Source: CAD feature listing. Evaluate the final solid. Frame: model axes, mm. A direction names the side the tool comes from. Give positions to 0.01 mm unless a question says otherwise; leave off trailing zeros. Loops run counter-clockwise (first coordinate to the right, second up) from the corner with the lowest first, then second, coordinate; pieces in that order, holes last. Notation, with made-up numbers: (79, 35) - (114, 35) arc R14 cw to (114, 57) - close; hole circle Ø7 at (1, 50.5). An arc over 180 degrees is marked (long way). Put each result on its own line as item: value.
```python
from build123d import *

# Parameters (mm, degrees)
F1_DEPTH = 152.4
F3_DEPTH = 151.892


with BuildPart() as f1:
    # F0 (on Top) → F1 (new body)
    with BuildSketch(Plane.XY):
        Polygon((127, 0), (0, 0), (-127, 0), (-127, -127), (127, -127), align=None)
        Polygon((-127, 0), (0, 0), (127, 0), (127, 127), (-127, 127), align=None)
    extrude(amount=F1_DEPTH)

    # F2 (on face) → F3 (cut)
    with BuildSketch(Plane.XY.offset(152.4)):
        Polygon((114.3, 0), (0, 0), (-114.3, 0), (-114.3, -114.3), (114.3, -114.3), align=None)
        Polygon((-114.3, 0), (0, 0), (114.3, 0), (114.3, 114.3), (-114.3, 114.3), align=None)
    extrude(amount=-F3_DEPTH, mode=Mode.SUBTRACT)


solid = f1.part
```
1) Access query for faces 5 (the flat face through (-2, -114.3, 78)), 6 (the flat face through (127, -2, 75)). Directions: +Z, -Z, +X, -X, +Y, -Y. A direction counts if a zero-diameter tool reaches every point of the face in a straight line with its end or side. Return the directions, or none.
Check result:
face 5: +Z
face 6: +Z, -Z, +X, +Y, -Y
2) Material intervals for line 1 along Y through (x, z) = (-16.5, 47.5); line 2 along Z through (x, y) = (59, 39.5), sorted ascending. Write a range as [from, to].
Check result:
line 1: [-127, -114.3], [114.3, 127]
line 2: [0, 0.51]
3) Section query B-B, the plane y = -11. Output: boundary loops of the cut face in (x, z), plus the area to 3 significant figures.
Check result:
outline: (-127, 0) - (127, 0) - (127, 152.4) - (114.3, 152.4) - (114.3, 0.51) - (-114.3, 0.51) - (-114.3, 152.4) - (-127, 152.4) - close
area: 3,990 mm²
4) Section query A-A, the plane z = 65. Output: boundary loops of the cut face in (x, y).
Check result:
outline: (-127, -127) - (127, -127) - (127, 127) - (-127, 127) - close; hole (-114.3, -114.3) - (114.3, -114.3) - (114.3, 114.3) - (-114.3, 114.3) - close
5) Mould query, pull axis Y, two halves, no side actions, for faces 1 (the flat face through (114.3, -2, 78)), 2 (the flat face through (2, 114.3, 78)), 3 (the flat face through (-2, -127, 75)), 4 (the flat face through (-127, 2, 75)). Classes: pulls with the +Y half, pulls with the -Y half, needs draft (parallel to the pull), parting line crosses it, or undercut.
Check result:
face 1: undercut
face 2: undercut
face 3: pulls with the -Y half
face 4: needs draft
6) Pin query (flat end, axial travel): P1, Ø4, axis at x = 33, y = -87, coming from the +Z side. Return the tip coordinate at first contact, or that it passes through.
Check result:
P1: z = 0.51
